For this review, take the finished solid that the model builds, in its own axes (mm). Face numbers are marked on the shaded views. A direction names the side the tool comes from. Coordinates: 2 decimals unless noted, no trailing zeros. Loops run counter-clockwise (first coordinate to the right, second up) from the corner with the lowest first, then second, coordinate; pieces in that order, holes last.
1. Clearance check with flat-ended pins moving along their axes: P1, Ø2, axis at x = 29, z = 10.5, coming from the +Y side; P2, Ø5, axis at x = 43, z = 22.5, coming from the -Y side; P3, Ø4, axis at x = -6.5, z = 5, coming from the -Y side; P4, Ø8, axis at x = 3.5, y = 36, coming from the -Z side. State where each tip first meets the part, or that it passes through.
2. Take a section at D-D, the plane y = -19. State the section outline as (x, z) points, then the cut area to 3 significant figures.
3. Take a section at A-A, the plane y = 0. State the section outline as (x, z) points.
4. Take a section at C-C, the plane z = 2. State the section outline as (x, y) points.
5. To check wall thickness, follow probe 1 along Y at (x, z) = (0, 2.3); probe 2 along Z at (x, y) = (65.5, 5); probe 3 along Y at (x, z) = (-35.5, 25.75). State the ranges of each line that lie inside material, in increasing order.
6. Mouldability with a two-part tool opening along X and no side actions: class the marked faces 1, 2 and 3 as pulls with the +X half, pulls with the -X half, needs draft (parallel to the pull), parting line crosses it, or undercut.
7. Machinability: for the marked faces 4, 5 and 6, which of the approach directions +Z, -Z, +X, -X, +Y, -Y give a long, thin tool a straight path to every point of the face, cutting with its end or side? Answer none if there is none.
```python
from build123d import *

# Parameters (mm, degrees)
SKETCH1_R           = 50
BOSS_EXTRUDE1_DEPTH = 20
SKETCH3_R           = 75
BOSS_EXTRUDE2_DEPTH = 10
SKETCH4_R           = 47.5
CUT_EXTRUDE3_DEPTH  = 25
SKETCH5_R           = 25
CUT_EXTRUDE4_DEPTH  = 25
SKETCH6_R           = 5
CUT_EXTRUDE5_DEPTH  = 25


with BuildPart() as part:
    # Sketch1 → Boss-Extrude1 (new body)
    with BuildSketch(Plane.XY):
        Circle(SKETCH1_R)
    extrude(amount=BOSS_EXTRUDE1_DEPTH)

    # Sketch3 → Boss-Extrude2 (add)
    with BuildSketch(Plane.XY.offset(20)):
        Circle(SKETCH3_R)
    extrude(amount=BOSS_EXTRUDE2_DEPTH)

    # Sketch4 → Cut-Extrude3 (cut)
    with BuildSketch(Plane.XY.offset(30)):
        Circle(SKETCH4_R)
    extrude(amount=-CUT_EXTRUDE3_DEPTH, mode=Mode.SUBTRACT)

    # Sketch5 → Cut-Extrude4 (cut)
    with BuildSketch(Plane.XY.offset(5)):
        Circle(SKETCH5_R)
    extrude(amount=-CUT_EXTRUDE4_DEPTH, mode=Mode.SUBTRACT)

    # Sketch6 → Cut-Extrude5 (cut)
    with BuildSketch(Plane.XY.offset(5)):
        with Locations((0, 35)):
            Circle(SKETCH6_R)
        with Locations((35, 0)):
            Circle(SKETCH6_R)
        with Locations((0, -35)):
            Circle(SKETCH6_R)
        with Locations((-35, 0)):
            Circle(SKETCH6_R)
    extrude(amount=-CUT_EXTRUDE5_DEPTH, mode=Mode.SUBTRACT)


solid = part.part
```
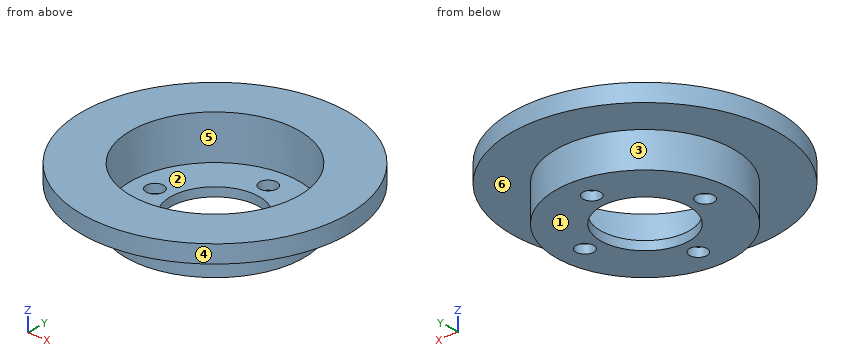
Results list:
1. P1: stops at y = 41.42
1. P2: stops at y = -63.12
1. P3: stops at y = -49.8
1. P4: stops at z = 0
2. outline: (-72.55, 20) - (-46.25, 20) - (-46.25, 0) - (-16.25, 0) - (-16.25, 5) - (-43.53, 5) - (-43.53, 30) - (-72.55, 30) - close; (16.25, 0) - (46.25, 0) - (46.25, 20) - (72.55, 20) - (72.55, 30) - (43.53, 30) - (43.53, 5) - (16.25, 5) - close
2. area: 962 mm2
3. outline: (-75, 20) - (-50, 20) - (-50, 0) - (-40, 0) - (-40, 5) - (-47.5, 5) - (-47.5, 30) - (-75, 30) - close; (-30, 0) - (-25, 0) - (-25, 5) - (-30, 5) - close; (25, 0) - (30, 0) - (30, 5) - (25, 5) - close; (40, 0) - (50, 0) - (50, 20) - (75, 20) - (75, 30) - (47.5, 30) - (47.5, 5) - (40, 5) - close
4. outline: circle Ø100 at (0, 0); hole circle Ø10 at (-35, 0); hole circle Ø50 at (0, 0); hole circle Ø10 at (0, -35); hole circle Ø10 at (0, 35); hole circle Ø10 at (35, 0)
5. probe 1: y = -50 to -40, -30 to -25, 25 to 30, 40 to 50
5. probe 2: z = 20 to 30
5. probe 3: y = -66.07 to -31.56, 31.56 to 66.07
6. face 1: needs draft
6. face 2: undercut
6. face 3: parting line crosses it
7. face 4: +Z, -Z
7. face 5: +Z
7. face 6: -Z
